Build history of the part. All positions in model axes, mm. Face numbers are marked on the shaded views. A direction names the side the tool comes from. Round coordinates to 2 decimals unless told otherwise and drop trailing zeros. Write each loop counter-clockwise with the first axis right and the second up, starting at its lowest first coordinate (ties: lowest second). Pieces come first, ordered by that corner, then holes. Notation, with made-up numbers: (88, 15) -> (135, 15) arc R29 cw to (135, 53) -> close; hole circle Ø4 at (30.5, 64.25). An arc over 180 degrees is marked (long way). Answer in a Markdown table with one row per item. Add a question column.
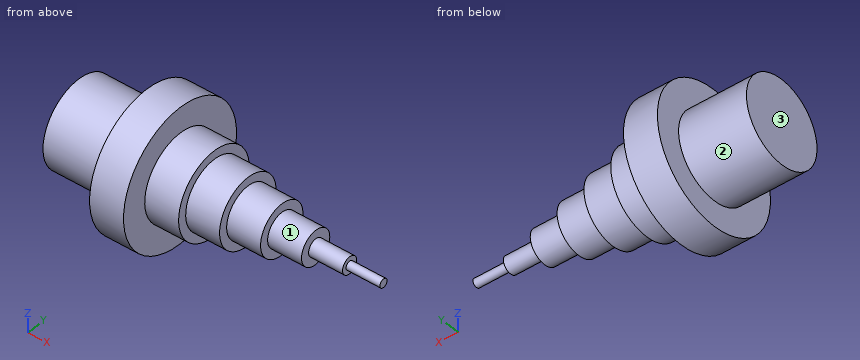
from build123d import *


with BuildPart() as part:
    # Sketch1 → Revolve4 (revolve)
    with BuildSketch(Plane.XY, mode=Mode.PRIVATE) as revolve4_sk:
        Polygon((-180, 0), (0, 0), (0, 2.5), (-20, 2.5), (-20, 5), (-40, 5), (-40, 10), (-60, 10), (-60, 15), (-80, 15), (-80, 20), (-100, 20), (-100, 25), (-120, 25), (-120, 40), (-140, 40), (-140, 25), (-180, 25), align=None)
    revolve(revolve4_sk.sketch.rotate(Axis((0, 0, 0), (-1, 0, 0)), 90), axis=Axis((0, 0, 0), (-1, 0, 0)))  # turned: the seam where the file's is


solid = part.part
(1) Drop flat-ended pins along their axis: P1, Ø15, axis at y = -6.5, z = 2, coming from the +X side; P2, Ø4, axis at y = -4, z = -12, coming from the +X side; P3, Ø4, axis at y = 24.5, z = 30.5, coming from the -X side; P4, Ø4, axis at x = -155.5, y = 19, coming from the -Z side. Give the stop position or say it passes through.
(2) Saw through at D-D (y = -22.5). List the corners of the cut face in (x, z), plus the area to 3 significant figures.
(3) Which spindle directions (+Z, -Z, +X, -X, +Y, -Y) get a long thin tool onto all of the face, cutting with end or side? Do the marked faces 1, 2 and 3. Say none if no direction does.
(4) Probe line 1 along X through (y, z) = (-16, 15.5); line 2 along X through (y, z) = (15.5, 30); line 3 along Y through (x, z) = (-171, -13.5). List the from-to ranges inside material, lowest first.
(5) Saw through at C-C (x = -124). List the corners of the cut face in (y, z), plus the area to 3 significant figures.
Answer sheet:
| question | item | result |
|---|---|---|
| 1 | P1 | stops at x = 0 |
| 1 | P2 | stops at x = -60 |
| 1 | P3 | stops at x = -140 |
| 1 | P4 | stops at z = -18.33 |
| 2 | outline | (-180, -10.9) -> (-140, -10.9) -> (-140, -33.07) -> (-120, -33.07) -> (-120, -10.9) -> (-100, -10.9) -> (-100, 10.9) -> (-120, 10.9) -> (-120, 33.07) -> (-140, 33.07) -> (-140, 10.9) -> (-180, 10.9) -> close |
| 2 | area | 2,630 mm² |
| 3 | face 1 | +X |
| 3 | face 2 | -X |
| 3 | face 3 | +Z, -Z, -X, +Y, -Y |
| 4 | line 1 | x = -180 to -100 |
| 4 | line 2 | x = -140 to -120 |
| 4 | line 3 | y = -21.04 to 21.04 |
| 5 | outline | circle Ø80 at (0, 0) |
| 5 | area | 5,030 mm² |
